Answer from the drawing. Dimensions are ordinates in mm from the lowest x, y and z of the part. A direction names the side the tool comes from. Give positions to 0.01 mm unless a question says otherwise; leave off trailing zeros. Loops run counter-clockwise (first coordinate to the right, second up) from the corner with the lowest first, then second, coordinate; pieces in that order, holes last. Notation, with made-up numbers: (3.5, 21.25) - (58.5, 21.25) arc R14 ccw to (58.5, 46.25) - close; hole circle Ø8 at (31.25, 27). An arc over 180 degrees is marked (long way). Answer as CSV lines item,"result". Start each with the question number.
1) Find the intervals of material crossed by line 1 along Z through (x, y) = (5, 5) (3 decimals); line 2 along X through (y, z) = (4.75, 5); line 3 along X through (y, z) = (4, 6), in increasing order.
2) A cutting plane is placed at C-C (y = 5.75). Determine the outline of the cut face in (x, z), and give its area (3 significant figures).
3) A cutting plane is placed at B-B (x = 6). Determine the outline of the cut face in (y, z).
4) Flat-ended cylindrical pins translate along their axes: pin 1 (0.8 mm diameter, centred on x = 2.5, z = 4, fed in from +Y); pin 2 (0.6 mm diameter, centred on y = 1.5, z = 3.5, fed in from -X) (3 decimals); pin 3 (0.8 mm diameter, centred on x = 5, y = 1.5, fed in from +Z) (3 decimals). Find the tip coordinate at first contact, or state that the pin passes through.
5) A cutting plane is placed at D-D (z = 5.5). Determine the outline of the cut face in (x, y).
6) For the marked faces 1 and 2, determine the directions among +Z, -Z, +X, -X, +Y, -Y from which every point of the face is accessible in a straight line to the end or side of a thin tool.
7) A cutting plane is placed at A-A (y = 4). Determine the outline of the cut face in (x, z) (3 decimals), and give its area (3 significant figures).
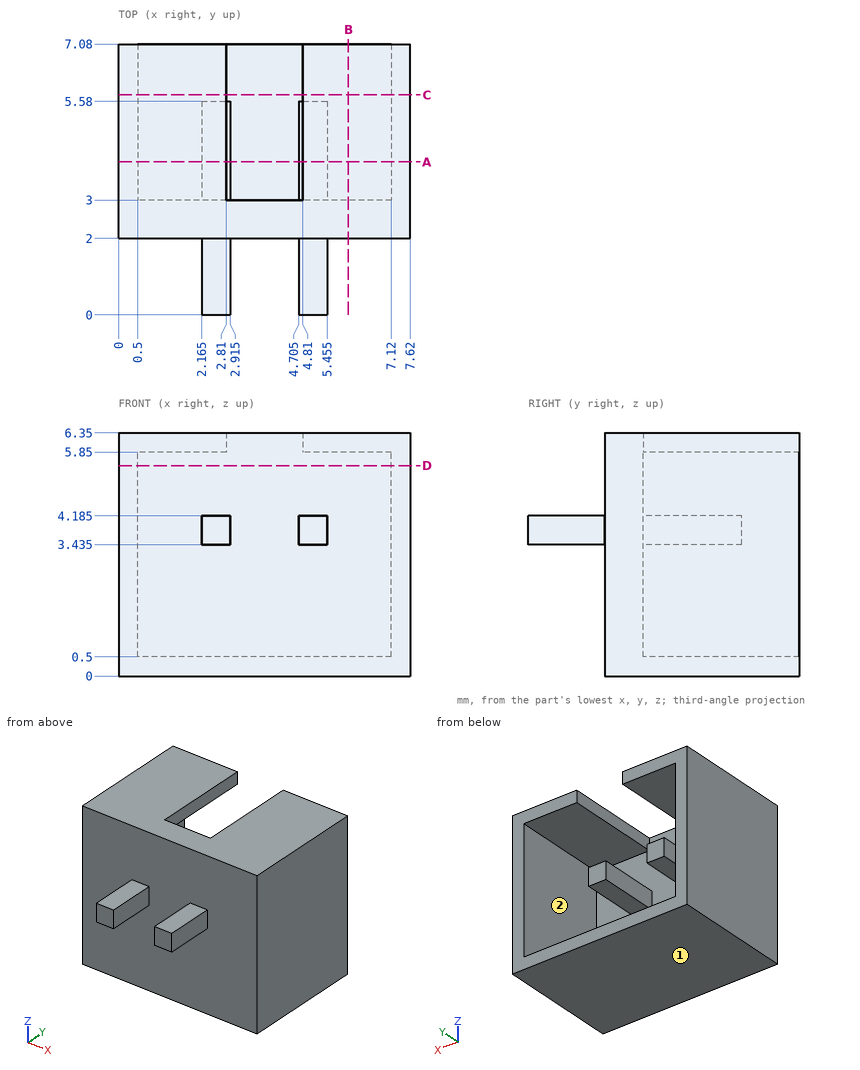
Ans:
1,line 1,"0 to 0.5, 3.435 to 4.185, 5.85 to 6.35"
1,line 2,"0 to 0.5, 7.12 to 7.62"
1,line 3,"0 to 2.81, 4.81 to 7.62"
2,outline,"(0, 0) - (7.62, 0) - (7.62, 6.35) - (4.81, 6.35) - (4.81, 5.85) - (7.12, 5.85) - (7.12, 0.5) - (0.5, 0.5) - (0.5, 5.85) - (2.81, 5.85) - (2.81, 6.35) - (0, 6.35) - close"
2,area,"12.0 mm2"
3,outline,"(2, 0) - (7.08, 0) - (7.08, 0.5) - (3, 0.5) - (3, 5.85) - (7.08, 5.85) - (7.08, 6.35) - (2, 6.35) - close"
4,pin 1,"y = 5.58"
4,pin 2,"x = 2.165"
4,pin 3,"z = 4.185"
5,outline,"(0, 2) - (7.62, 2) - (7.62, 7.08) - (7.12, 7.08) - (7.12, 3) - (0.5, 3) - (0.5, 7.08) - (0, 7.08) - close"
6,face 1,"-Z, +X, -X, +Y, -Y"
6,face 2,"+Y"
7,outline,"(0, 0) - (7.62, 0) - (7.62, 6.35) - (4.81, 6.35) - (4.81, 5.85) - (7.12, 5.85) - (7.12, 0.5) - (0.5, 0.5) - (0.5, 5.85) - (2.81, 5.85) - (2.81, 6.35) - (0, 6.35) - close; (2.165, 3.435) - (2.915, 3.435) - (2.915, 4.185) - (2.165, 4.185) - close; (4.705, 3.435) - (5.455, 3.435) - (5.455, 4.185) - (4.705, 4.185) - close"
7,area,"13.1 mm2"
